from build123d import *

# Parameters (mm, degrees)
SKETCH1_W           = 560
SKETCH1_H           = 560
BOSS_EXTRUDE1_DEPTH = 5
SKETCH2_W           = 418.578643762
SKETCH2_H           = 418.578643762
SKETCH2_W_2         = 408.578643762
SKETCH2_H_2         = 408.578643762
BOSS_EXTRUDE2_DEPTH = 45
SKETCH3_R           = 3
CUT_EXTRUDE1_DEPTH  = 5
FILLET1_R           = 5
FILLET2_R           = 2.5
FILLET3_R           = 2.5


with BuildPart() as part:
    # Sketch1 → Boss-Extrude1 (new body)
    with BuildSketch(Plane(origin=(0, 0, 0), x_dir=(1, 0, 0), z_dir=(0, 1, 0))):
        Rectangle(SKETCH1_W, SKETCH1_H)
    extrude(amount=BOSS_EXTRUDE1_DEPTH)

    # Sketch2 → Boss-Extrude2 (add)
    with BuildSketch(Plane(origin=(0, 5, 0), x_dir=(1, 0, 0), z_dir=(0, 1, 0))):
        Rectangle(SKETCH2_W, SKETCH2_H)
        Rectangle(SKETCH2_W_2, SKETCH2_H_2, mode=Mode.SUBTRACT)
    extrude(amount=BOSS_EXTRUDE2_DEPTH)

    # Sketch3 → Cut-Extrude1 (cut)
    with BuildSketch(Plane(origin=(0, 5, 0), x_dir=(1, 0, 0), z_dir=(0, 1, 0))):
        with Locations(Location((7.5, 52.990381057, 0), (0, 0, 270))):
            Circle(SKETCH3_R)
        with Locations(Location((0, 40, 0), (0, 0, 270))):
            Circle(SKETCH3_R)
        with Locations(Location((-7.5, 52.990381057, 0), (0, 0, 270))):
            Circle(SKETCH3_R)
    extrude(amount=-CUT_EXTRUDE1_DEPTH, mode=Mode.SUBTRACT)

    # Fillet1
    fillet1_edges = [part.edges().sort_by_distance(p)[0] for p in [
        (0, 5, -204.289321881),
        (204.289321881, 5, 0),
        (-209.289321881, 5, 0),
        (0, 5, 209.289321881),
        (209.289321881, 5, 0),
        (0, 5, -209.289321881),
        (-204.289321881, 5, 0),
        (0, 5, 204.289321881),
    ]]
    fillet(fillet1_edges, radius=FILLET1_R)

    # Fillet2
    fillet2_edges = [part.edges().sort_by_distance(p)[0] for p in [
        (0, 50, 204.289321881),
        (209.289321881, 50, 0),
        (0, 50, -209.289321881),
        (-204.289321881, 50, 0),
        (-209.289321881, 50, 0),
        (0, 50, 209.289321881),
        (0, 50, -204.289321881),
        (204.289321881, 50, 0),
    ]]
    fillet(fillet2_edges, radius=FILLET2_R - 0.0001)  # a hair under: the kernel refuses the full size

    # Fillet3
    fillet3_edges = [part.edges().sort_by_distance(p)[0] for p in [
        (-280, 5, 0),
        (0, 5, 280),
        (280, 5, 0),
        (0, 0, 280),
        (-280, 0, 0),
        (0, 0, -280),
        (280, 0, 0),
        (280, 2.5, 280),
        (-280, 2.5, 280),
        (-280, 2.5, -280),
        (280, 2.5, -280),
        (0, 5, -280),
    ]]
    fillet(fillet3_edges, radius=FILLET3_R - 0.0001)  # a hair under: the kernel refuses the full size


solid = part.part
Could you check a few things on this model? Use its own coordinates, in mm. A direction names the side the tool comes from. Give positions to 0.01 mm unless a question says otherwise; leave off trailing zeros. Write each loop counter-clockwise with the first axis right and the second up, starting at its lowest first coordinate (ties: lowest second). Pieces come first, ordered by that corner, then holes. Notation, with made-up numbers: (52.5, -24) - (81.5, -24) arc R29 cw to (81.5, 14) - close; hole circle Ø5 at (77, 55.25). An arc over 180 degrees is marked (long way). Use CSV: the item, a comma, the result in double quotes. Start each with the question number.
Item 1: If we mould it in two halves opening along Z, with no side actions, what happens to faces 1 (the face through (-4, 0, -4)), 2 (the face through (204.289, 28, 3)), 3 (the face through (-3, 28, -209.289))? For each: pulls with the +Z half, pulls with the -Z half, needs draft (parallel to the pull), parting line crosses it, or undercut.
Item 2: I want a section at B-B, the plane y = 41. Please give me the cut outline in (x, z).
Item 3: If I drill on line 1 along Z through (x, y) = (53, 35.5); line 2 along Z through (x, y) = (7, 3), over which ranges is the centre line in solid material (lowest first)?
Item 4: I'm going to push flat-ended pins straight in: pin 1 (19 mm diameter, centred on x = -16.5, y = 21, fed in from -Z); pin 2 (5 mm diameter, centred on x = 36.5, y = 9, fed in from +Z); pin 3 (5.5 mm diameter, centred on x = 7.5, z = -52.99, fed in from +Y); pin 4 (5 mm diameter, centred on x = -16.5, z = 49, fed in from +Y). Where does each tip first touch, or does it pass through?
Item 5: For faces 4 (the face through (-209.289, 28, 3)), 5 (the face through (-3, 28, 209.289)), 6 (the face through (-3, 28, -204.289)), which set-ups out of +Z, -Z, +X, -X, +Y, -Y let a thin tool reach every point of the face, with its end or its side?
Findings:
1,face 1,"needs draft"
1,face 2,"undercut"
1,face 3,"pulls with the -Z half"
2,outline,"(-209.29, -209.29) - (209.29, -209.29) - (209.29, 209.29) - (-209.29, 209.29) - close; hole (-204.29, -204.29) - (204.29, -204.29) - (204.29, 204.29) - (-204.29, 204.29) - close"
3,line 1,"z = -209.29 to -204.29, 204.29 to 209.29"
3,line 2,"z = -279.95 to -55.95, -50.03 to 279.95"
4,pin 1,"stops at z = -209.29"
4,pin 2,"stops at z = 210.72"
4,pin 3,"passes through"
4,pin 4,"stops at y = 5"
5,face 4,"+Z, -Z, -X, +Y"
5,face 5,"+Z, +X, -X, +Y"
5,face 6,"+Y"
